The drawing under review shows one solid part. Ordinate dimensions are in mm from its lowest x, y, z. Round coordinates to 2 decimals unless told otherwise and drop trailing zeros. Write each loop counter-clockwise with the first axis right and the second up, starting at its lowest first coordinate (ties: lowest second). Pieces come first, ordered by that corner, then holes.
Item 1: Add section C-C (z = 30.2). Give the boundary of the cut face in (x, y).
Item 2: To check wall thickness, follow L1, parallel to Z at x = 4.4, y = 1.2; L2, parallel to X at y = 1.1, z = 30.2; L3, parallel to Z at x = 27.5, y = 1.1. State the ranges of each line that lie inside material, in increasing order.
Item 3: Add section D-D (y = 0.5). Give the boundary of the cut face in (x, z), plus the area to 3 significant figures.
Item 4: Add section A-A (x = 7). Give the boundary of the cut face in (y, z).
Item 5: Add section B-B (x = 27.5). Give the boundary of the cut face in (y, z).
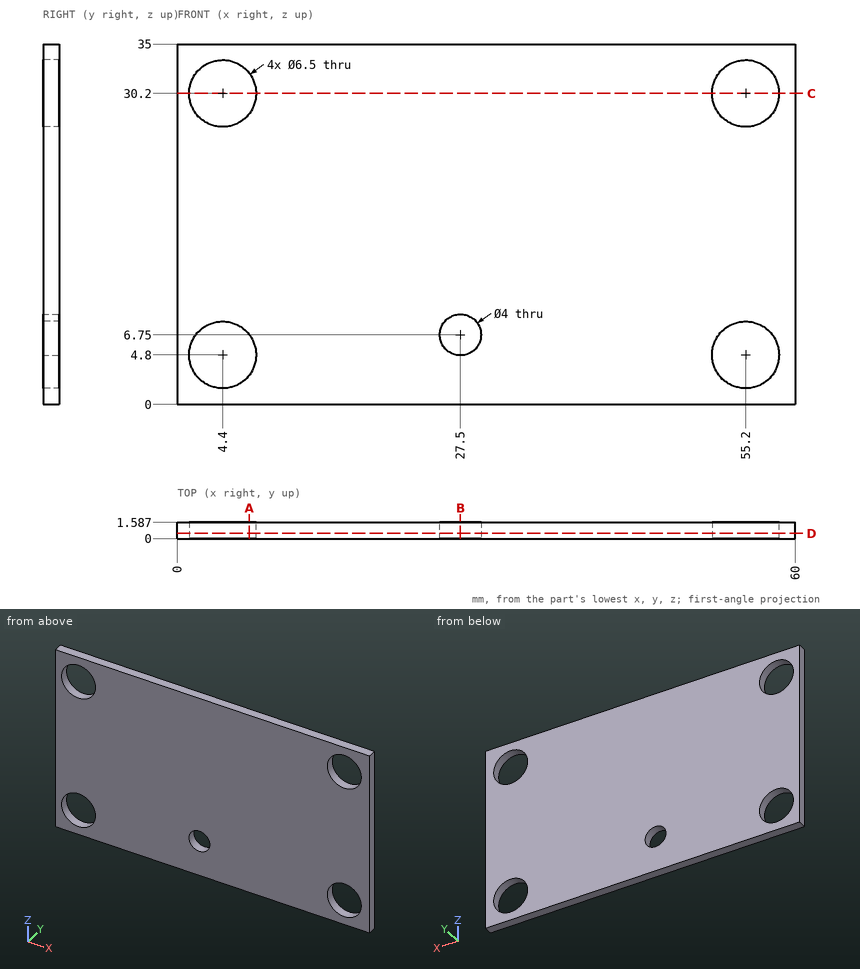
Numbers:
1. outline: (0, 0) - (1.15, 0) - (1.15, 1.59) - (0, 1.59) - close; (7.65, 0) - (51.95, 0) - (51.95, 1.59) - (7.65, 1.59) - close; (58.45, 0) - (60, 0) - (60, 1.59) - (58.45, 1.59) - close
2. L1: z = 0 to 1.55, 8.05 to 26.95, 33.45 to 35
2. L2: x = 0 to 1.15, 7.65 to 51.95, 58.45 to 60
2. L3: z = 0 to 4.75, 8.75 to 35
3. outline: (0, 0) - (60, 0) - (60, 35) - (0, 35) - close; hole circle Ø6.5 at (4.4, 4.8); hole circle Ø6.5 at (4.4, 30.2); hole circle Ø4 at (27.5, 6.75); hole circle Ø6.5 at (55.2, 4.8); hole circle Ø6.5 at (55.2, 30.2)
3. area: 1,950 mm2
4. outline: (0, 0) - (1.59, 0) - (1.59, 2.85) - (0, 2.85) - close; (0, 6.75) - (1.59, 6.75) - (1.59, 28.25) - (0, 28.25) - close; (0, 32.15) - (1.59, 32.15) - (1.59, 35) - (0, 35) - close
5. outline: (0, 0) - (1.59, 0) - (1.59, 4.75) - (0, 4.75) - close; (0, 8.75) - (1.59, 8.75) - (1.59, 35) - (0, 35) - close
